Solid Edge part; units mm, degrees
sketch "Sketch1" plane through (0, 0, 0) normal (0, 0, 1) x (1, 0, 0)
  circle A0 centre (0, 0) radius 1.5
extrude "Protrusion1" add sketch "Sketch1" along normal blind 30
sketch "Sketch2" plane through (0, 0, 30) normal (0, 0, 1) x (1, 0, 0)
  circle A0 centre (0, 0) radius 3
extrude "ExtrudedProtrusion_2" add sketch "Sketch2" along normal blind 1.75
chamfer "Chamfer_1" distance 1.75 angle 45 1 edges at (-3, 0, 30)
sketch "Sketch3" plane through (0, 0, 31.75) normal (0, 0, 1) x (0, 1, 0)
  line L0 (0.8978, -1.555) -> (1.7956, 0)
  line L1 (1.7956, 0) -> (0.8978, 1.555)
  line L2 (0.8978, 1.555) -> (-0.8978, 1.555)
  line L3 (-0.8978, 1.555) -> (-1.7956, 0)
  line L4 (-1.7956, 0) -> (-0.8978, -1.555)
  line L5 (-0.8978, -1.555) -> (0.8978, -1.555)
extrude "ExtrudedCutout_1" cut sketch "Sketch3" against normal blind 1
sketch "Sketch4" plane through (0, 0, 0) normal (0, 0, -1) x (0, 1, 0)
  circle A0 centre (0, 0) radius 1.9215
extrude "ExtrudedCutout_2" cut sketch "Sketch4" against normal blind 25.75
revolve "RevolvedCutout1" [suppressed]
fillet "Round_1" [suppressed]
properties material "Iron, grey cast type 20"
Could you check a few things on this model? Use its own coordinates, in mm. A direction names the side the tool comes from. Round coordinates to 2 decimals unless told otherwise and drop trailing zeros. Loops run counter-clockwise (first coordinate to the right, second up) from the corner with the lowest first, then second, coordinate; pieces in that order, holes last.
Q1. On a 3-axis mill with a long thin cutter (end or side, diameter ignored), from which of +Z, -Z, +X, -X, +Y, -Y can I reach the whole of each face in a straight line? I mean faces 5 (the flat face through (0, 0, 25.75)), 6 (the flat face through (0.79, 1.34, 31.26)). Say none if no direction works.
Q2. I want a section at B-B (y = 0). Write out the boundary of the cut face in (x, z) (3 decimals), and give its area (3 significant figures).
Q3. I want a section at C-C (z = 29.6). Write out the boundary of the cut face in (x, y), and give its area (3 significant figures).
Q4. For P1, Ø1.5, axis at y = -2.5, z = 29.5, coming from the +X side; P2, Ø1.5, axis at x = -2, z = 30.5, coming from the +Y side; P3, Ø1.1, axis at y = -0.5, z = 31, coming from the +X side, each with a flat end and sliding along its axis, tell me the tip position at first contact or that it passes through.
Q5. I want a section at A-A (z = 31.15). Write out the boundary of the cut face in (x, y) (3 decimals), and give its area (3 significant figures).
Q6. Thinking about a two-plate mould opening in X: for faces 1 (the flat face through (0, 0, 30.75)), 2 (the flat face through (1.3, -1.3, 31.75)), 3 (the cylindrical face through (-1.5, -0.07, 27.97)), 4 (the flat face through (-0.77, 1.35, 31.26)), which applies, pulls with the +X half, pulls with the -X half, needs draft (parallel to the pull), parting line crosses it, or undercut?
Q7. Please list where these lines run through material, in increasing order: L1, parallel to X at y = -0.1, z = 31.45 (3 decimals); L2, parallel to Z at x = -1.2, y = 0.45; L3, parallel to X at y = 1.45, z = 31.25.
Answer below:
1. face 5: -Z, +X, -X, +Y, -Y
1. face 6: +Z
2. outline: (-3, 31.75) - (-1.5, 30.25) - (-1.5, 25.75) - (1.5, 25.75) - (1.5, 30.25) - (3, 31.75) - (1.555, 31.75) - (1.555, 30.75) - (-1.555, 30.75) - (-1.555, 31.75) - close
2. area: 17.1 mm2
3. outline: circle Ø3 at (0, 0)
3. area: 7.07 mm2
4. P1: passes through
4. P2: stops at y = 1.77
4. P3: stops at x = 2.76
5. outline: circle Ø4.8 at (0, 0); hole (-1.555, -0.898) - (0, -1.796) - (1.555, -0.898) - (1.555, 0.898) - (0, 1.796) - (-1.555, 0.898) - close
5. area: 9.72 mm2
6. face 1: undercut
6. face 2: needs draft
6. face 3: parting line crosses it
6. face 4: undercut
7. L1: x = -2.698 to -1.555, 1.555 to 2.698
7. L2: z = 25.75 to 30.75
7. L3: x = -2.04 to -0.6, 0.6 to 2.04
